Read the model definition and answer for the solid it produces. Units are mm, in the model's axes. Coordinates: 2 decimals unless noted, no trailing zeros. Write each loop counter-clockwise with the first axis right and the second up, starting at its lowest first coordinate (ties: lowest second). Pieces come first, ordered by that corner, then holes.
(1) Find the intervals of material crossed by probe 1 along X at (y, z) = (60.5, 26); probe 2 along X at (y, z) = (8.5, 44.5); probe 3 along Y at (x, z) = (-142.5, 35.5), in increasing order.
(2) Section A-A on z = 28 is taken. Write down the section's boundary in (x, y).
(3) Section B-B on x = -29 is taken. Write down the section's boundary in (y, z), then the cut area to 3 significant figures.
(4) Given pin 1 (8 mm diameter, centred on y = 25, z = 13.5, fed in from +X); pin 2 (5 mm diameter, centred on x = -39, z = 45.5, fed in from +Y); pin 3 (8 mm diameter, centred on x = -65, z = 32, fed in from +Y), each flat-ended and moving along its own axis, determine where each tip first touches the part or whether it passes through.
(5) Section C-C on y = 37.5 is taken. Write down the section's boundary in (x, z), then the cut area to 3 significant figures.
from build123d import *

# Parameters (mm, degrees)
EXTRUDE_1_DEPTH = 30
FILLET_1_R      = 10
SCALE_1_SCALE   = 2


with BuildPart() as part:
    # 草图1 → 凸台-拉伸1 (new body)
    with BuildSketch(Plane.XY):
        Polygon((-90, 0), (0, 0), (-44.31605129, 77.54338676), align=None)
    extrude(amount=EXTRUDE_1_DEPTH)

    # 圆角1
    fillet_1_edges = [part.edges().sort_by_distance(p)[0] for p in [
        (0, 0, 15),
        (-90, 0, 15),
        (-44.31605129, 77.54338676, 15),
    ]]
    fillet(fillet_1_edges, radius=FILLET_1_R)


with BuildPart() as part_1:
    # 缩放比例1: scaled about (0, 0, 0)
    add(part.part.scale(SCALE_1_SCALE))


solid = part_1.part
Response:
1. probe 1: x = -144.36 to -34.58
1. probe 2: x = -161.37 to -18.1
1. probe 3: y = 0 to 63.65
2. outline: (-162.24, 30.15) arc R20 ccw to (-145, 0) - (-34.47, 0) arc R20 ccw to (-17.1, 29.92) - (-71.53, 125.16) arc R20 ccw to (-106.13, 125.39) - close
3. outline: (0.76, 0) - (50.74, 0) - (50.74, 60) - (0.76, 60) - close
3. area: 3,000 mm2
4. pin 1: stops at x = -14.49
4. pin 2: stops at y = 72.62
4. pin 3: stops at y = 120.73
5. outline: (-157.91, 0) - (-21.43, 0) - (-21.43, 60) - (-157.91, 60) - close
5. area: 8,190 mm2
